For this review, use the dimensioned drawing (mm, ordinates from the lowest corner) and the shaded views. A direction names the side the tool comes from. Give positions to 0.01 mm unless a question says otherwise; leave off trailing zeros. Loops run counter-clockwise (first coordinate to the right, second up) from the corner with the lowest first, then second, coordinate; pieces in that order, holes last. Notation, with made-up numbers: M -6,33 L -2,33 A15 cw -2,58 Z; hole C -0.75,67 d2. An arc over 180 degrees is marked long. Use a Markdown table: item, result. Add a question column.
(1) Add section B-B, the plane x = 484.5. Give the boundary of the cut face in (y, z).
(2) Draft analysis for pull direction X (two halves, no side actions). For the marked faces 1, 2, 3 and 4, state which applies: pulls with the +X half, pulls with the -X half, needs draft (parallel to the pull), parting line crosses it, or undercut.
(3) For probe 1 along X at (y, z) = (671.5, 578.5); probe 2 along Z at (x, y) = (274.5, 317.5), list the stretches that pass through material, from the lowest coordinate up.
(4) For the marked faces 5 and 6, list the 3-axis set-ups (+Z, -Z, +X, -X, +Y, -Y) from which the entire face can be reached by the end or side of a thin tool; tool diameter is ignored.
(5) Add section A-A, the plane y = 174.5. Give the boundary of the cut face in (x, z), then the cut area to 3 significant figures.
(6) Add section C-C, the plane z = 378.5. Give the boundary of the cut face in (x, y).
(7) Add section D-D, the plane y = 63.5. Give the boundary of the cut face in (x, z).
(8) Insertion check: pin 1 Ø2 at (x, y) = (933, 501) entering from -Z. The pin has a flat end and moves straight along its axis. Give the tip position at first contact, or say it passes through.
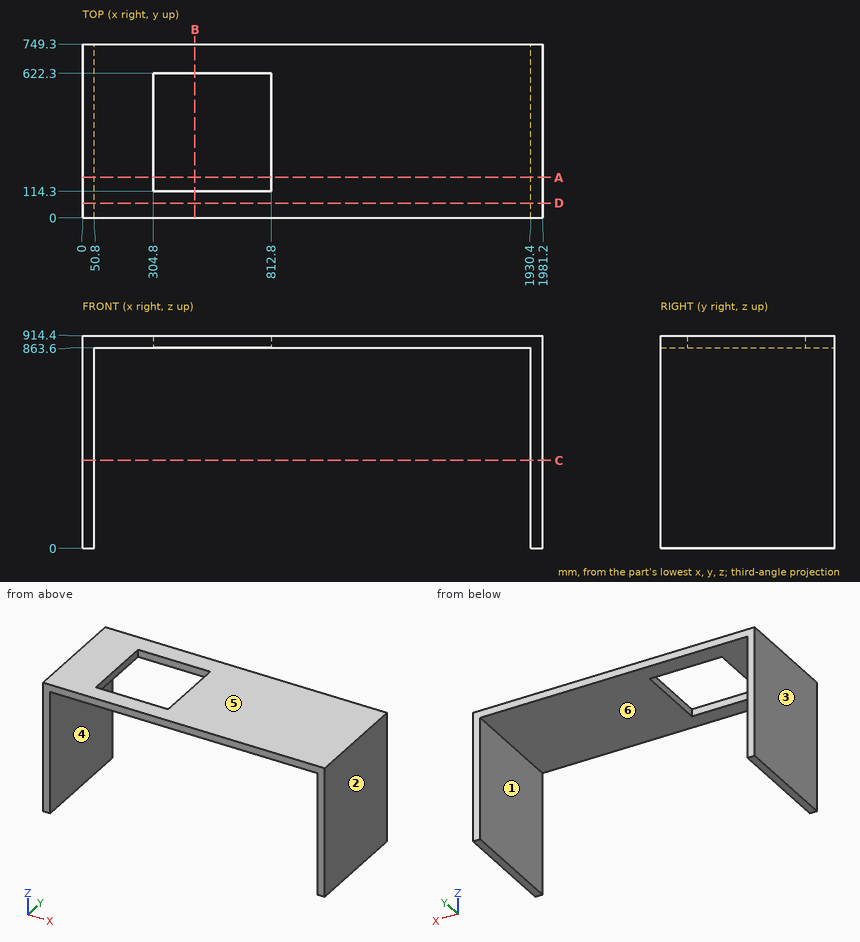
Established:
| question | item | result |
|---|---|---|
| 1 | outline | M 0,863.6 L 114.3,863.6 L 114.3,914.4 L 0,914.4 Z; M 622.3,863.6 L 749.3,863.6 L 749.3,914.4 L 622.3,914.4 Z |
| 2 | face 1 | undercut |
| 2 | face 2 | pulls with the +X half |
| 2 | face 3 | pulls with the -X half |
| 2 | face 4 | undercut |
| 3 | probe 1 | 0 to 50.8, 1930.4 to 1981.2 |
| 3 | probe 2 | 863.6 to 914.4 |
| 4 | face 5 | +Z, +X, -X, +Y, -Y |
| 4 | face 6 | -Z, +Y, -Y |
| 5 | outline | M 0,0 L 50.8,0 L 50.8,863.6 L 304.8,863.6 L 304.8,914.4 L 0,914.4 Z; M 812.8,863.6 L 1930.4,863.6 L 1930.4,0 L 1981.2,0 L 1981.2,914.4 L 812.8,914.4 Z |
| 5 | area | 163,000 mm^2 |
| 6 | outline | M 0,0 L 50.8,0 L 50.8,749.3 L 0,749.3 Z; M 1930.4,0 L 1981.2,0 L 1981.2,749.3 L 1930.4,749.3 Z |
| 7 | outline | M 0,0 L 50.8,0 L 50.8,863.6 L 1930.4,863.6 L 1930.4,0 L 1981.2,0 L 1981.2,914.4 L 0,914.4 Z |
| 8 | pin 1 | z = 863.6 |
